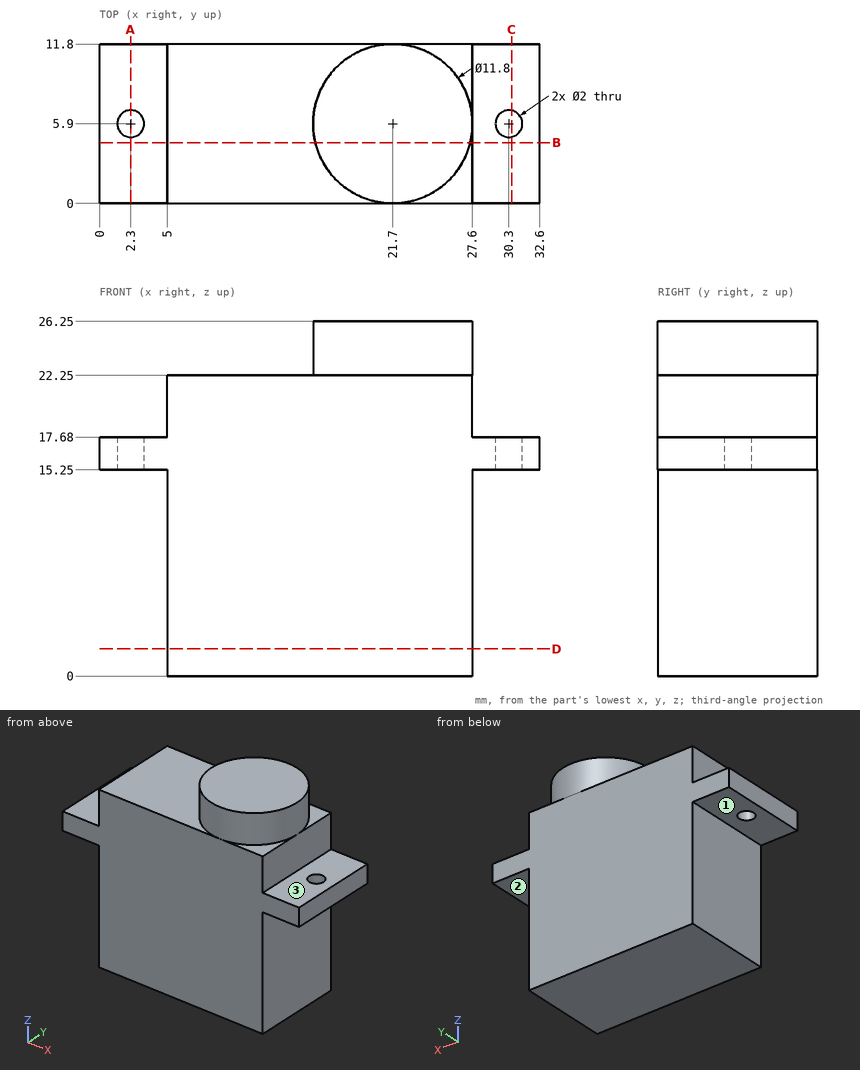
For this review, use the dimensioned drawing (mm, ordinates from the lowest corner) and the shaded views. A direction names the side the tool comes from. Coordinates: 2 decimals unless noted, no trailing zeros. Loops run counter-clockwise (first coordinate to the right, second up) from the corner with the lowest first, then second, coordinate; pieces in that order, holes last. Notation, with made-up numbers: (-21.75, 76.5) -> (-16.75, 76.5) arc R13 ccw to (-16.75, 84.5) -> close; hole circle Ø10 at (40, 81.5). An arc over 180 degrees is marked (long way). Write each question's results on one line, items separated by ' | '.
Q1. For pin 1 Ø2.5 at (x, y) = (31, 6.5) entering from -Z; pin 2 Ø1 at (x, z) = (28.5, 4) entering from -Y; pin 3 Ø1.5 at (y, z) = (1.5, 3.5) entering from -X; pin 4 Ø1.4 at (y, z) = (4, 19) entering from +X, all flat-tipped, find the tip position at first contact; note any pin that passes through.
Taken from the geometry:
pin 1: z = 15.25 | pin 2: through | pin 3: x = 5 | pin 4: x = 27.6
Q2. Machinability: for the marked faces 1, 2 and 3, which of the approach directions +Z, -Z, +X, -X, +Y, -Y give a long, thin tool a straight path to every point of the face, cutting with its end or side? Answer none if there is none.
Taken from the geometry:
face 1: -Z, -X, +Y, -Y | face 2: -Z, +X, +Y, -Y | face 3: +Z, +X, +Y, -Y
Q3. Add section B-B, the plane y = 4.5. State the section outline as (x, z) points.
Taken from the geometry:
outline: (0, 15.25) -> (5, 15.25) -> (5, 0) -> (27.6, 0) -> (27.6, 15.25) -> (32.6, 15.25) -> (32.6, 17.68) -> (27.6, 17.68) -> (27.6, 22.25) -> (27.43, 22.25) -> (27.43, 26.25) -> (15.97, 26.25) -> (15.97, 22.25) -> (5, 22.25) -> (5, 17.68) -> (0, 17.68) -> close
Q4. Add section C-C, the plane x = 30.5. State the section outline as (y, z) points, then the cut area to 3 significant figures.
Taken from the geometry:
outline: (0, 15.25) -> (4.92, 15.25) -> (4.92, 17.68) -> (0, 17.68) -> close; (6.88, 15.25) -> (11.8, 15.25) -> (11.8, 17.68) -> (6.88, 17.68) -> close | area: 23.9 mm²
Q5. To check wall thickness, follow line 1 along Y through (x, z) = (2.3, 16.7); line 2 along Z through (x, y) = (4, 5.75); line 3 along X through (y, z) = (4.25, 8.5). State the ranges of each line that lie inside material, in increasing order. Write a range as [from, to].
Taken from the geometry:
line 1: [0, 4.9], [6.9, 11.8] | line 2: [15.25, 17.68] | line 3: [5, 27.6]
Q6. Add section D-D, the plane z = 2. State the section outline as (x, y) points.
Taken from the geometry:
outline: (5, 0) -> (27.6, 0) -> (27.6, 11.8) -> (5, 11.8) -> close
Q7. Add section A-A, the plane x = 2.3. State the section outline as (y, z) points, then the cut area to 3 significant figures.
Taken from the geometry:
outline: (0, 15.25) -> (4.9, 15.25) -> (4.9, 17.68) -> (0, 17.68) -> close; (6.9, 15.25) -> (11.8, 15.25) -> (11.8, 17.68) -> (6.9, 17.68) -> close | area: 23.8 mm²
